Could you check a few things on this model? Use its own coordinates, in mm. A direction names the side the tool comes from. Coordinates: 2 decimals unless noted, no trailing zeros. Order: outer loops, then holes, each group sorted by start corner. A loop starts at its lowest first (then second) coordinate and runs counter-clockwise, first axis right, second up.
```python
from build123d import *

# Parameters (mm, degrees)
F0_R     = 5
F1_DEPTH = 44
F2_R     = 2.5
F3_DEPTH = 10
F4_SIZE  = 1
F5_R     = 3


with BuildPart() as f1:
    # F0 (on Right) → F1 (new body)
    with BuildSketch(Plane.YZ):
        Circle(F0_R)
    extrude(amount=F1_DEPTH)

    # F2 (on face) → F3 (join)
    with BuildSketch(Plane(origin=(0, 0, 0), x_dir=(0, -1, 0), z_dir=(-1, 0, 0))):
        Circle(F2_R)
    extrude(amount=F3_DEPTH)

    # F4
    f4_edges = [f1.edges().sort_by_distance(p)[0] for p in [
        (-10, 2.5, 0),
    ]]
    chamfer(f4_edges, length=F4_SIZE)

    # F5
    f5_edges = [f1.edges().sort_by_distance(p)[0] for p in [
        (44, -5, 0),
    ]]
    fillet(f5_edges, radius=F5_R)


solid = f1.part
```
Item 1: I need wall thicknesses on line 1 (Y direction, x = 39, z = -0.25); line 2 (Y direction, x = -0.5, z = -2); line 3 (X direction, y = -2, z = 3.75). Which ranges of each line are inside material? Lowest first, please.
Item 2: For pin 1 Ø4 at (x, y) = (34.5, 1.5) entering from +Z; pin 2 Ø2 at (y, z) = (-3.5, 3) entering from -X; pin 3 Ø1.5 at (x, z) = (9.5, 3.5) entering from -Y; pin 4 Ø3 at (x, y) = (35.5, -3.5) entering from -Z, each with a flat end and sliding along its axis, tell me the tip position at first contact or that it passes through.
Item 3: Suppose I cut it at A-A (x = 9). List the corners of the cut face in (y, z) for me.
Item 4: Which directions (+Z, -Z, +X, -X, +Y, -Y) give clear straight access to the entire face, cutting with the end or side of a thin tool? Please do faces 1 (the face through (-4.44, 0.54, -2.44)), 2 (the face through (-10, 0, 0)).
Geometry results:
1. line 1: y = -4.99 to 4.99
1. line 2: y = -1.5 to 1.5
1. line 3: x = 0 to 42.98
2. pin 1: stops at z = 5
2. pin 2: stops at x = 0
2. pin 3: stops at y = -4.18
2. pin 4: stops at z = -4.58
3. outline: circle Ø10 at (0, 0)
4. face 1: -X
4. face 2: +Z, -Z, -X, +Y, -Y
